from build123d import *

# Parameters (mm, degrees)
BOSS_EXTRUDE1_DEPTH      = 97
BOSS_EXTRUDE1_DEPTH_BACK = 64
SKETCH6_R                = 3
CUT_EXTRUDE1_DEPTH       = 10
SKETCH8_R                = 3
CUT_EXTRUDE3_DEPTH       = 10


with BuildPart() as part:
    # Sketch3 → Boss-Extrude1 (new, two sides: drawn at the far end of the back side and taken through both)
    with BuildSketch(Plane(origin=(-16.16759993, 0, 0), x_dir=(0, 0, -1), z_dir=(1, 0, 0)).offset(-BOSS_EXTRUDE1_DEPTH_BACK)):
        Polygon((746.208968128, 603.456840762), (886.208968128, 603.456840762), (949.708968128, 493.471614481), (923.661741478, 345.75045153), (946.661741478, 345.75045153), (946.661741478, 347.02045153), (925.175268541, 347.02045153), (951.03994149, 493.706300996), (886.94220297, 604.726840762), (745.475733286, 604.726840762), (681.358982713, 493.673371154), (730.060945884, 282.721992649), (731.298395866, 283.007680488), (682.708968128, 493.471614481), align=None)
    extrude(amount=BOSS_EXTRUDE1_DEPTH + BOSS_EXTRUDE1_DEPTH_BACK)

    # Sketch6 → Cut-Extrude1 (cut)
    with BuildSketch(Plane(origin=(0, 347.02045153, 0), x_dir=(1, 0, 0), z_dir=(0, 1, 0))):
        with Locations(Location((-69.5, 935.918505009, 0), (0, 0, 180))):
            Circle(SKETCH6_R)
        with Locations(Location((69.000000001, 935.918505009, 0), (0, 0, 180))):
            Circle(SKETCH6_R)
    extrude(amount=-CUT_EXTRUDE1_DEPTH, mode=Mode.SUBTRACT)

    # Sketch8 → Cut-Extrude3 (cut)
    with BuildSketch(Plane(origin=(0, 174.325401486, -755.08627081), x_dir=(1, 0, 0), z_dir=(0, -0.22495105434386187, 0.9743700647852359))):
        with Locations(Location((69, 160.202749263, 0), (0, 0, 270))):
            Circle(SKETCH8_R)
        with Locations(Location((-69.5, 160.49556469, 0), (0, 0, 270))):
            Circle(SKETCH8_R)
    extrude(amount=-CUT_EXTRUDE3_DEPTH, mode=Mode.SUBTRACT)


solid = part.part
Model file for the job. Use its own axes, mm. A direction names the side the tool comes from. Coordinates: 2 decimals unless noted, no trailing zeros. Loops run counter-clockwise (first coordinate to the right, second up) from the corner with the lowest first, then second, coordinate; pieces in that order, holes last. Notation, with made-up numbers: (62, 41) -> (111, 41) arc R35 cw to (111, 76) -> close; hole circle Ø6 at (78, -17.75). An arc over 180 degrees is marked (long way). Use one line per item in the form item = value. Start each with the question number.
(1) Cut at C-C on x = 22. Give the cut face in (y, z).
(2) Tool access for faces 1 (the flat face through (-1, 603.457, -815)), 2 (the flat face through (-1, 347.02, -936)), 3 (the flat face through (-0.79, 547.69, -714.01)): list every direction of +Z, -Z, +X, -X, +Y, -Y with a clear straight run to the whole face (end or side of a thin tool).
(3) Cut at B-B on y = 400.5. Give the cut face in (x, z), and give its area (3 significant figures).
(4) Cut at A-A on z = -700.5. Give the cut face in (x, y), and give its area (3 significant figures).
(5) Pull direction Z, two halves, no side cores. Call faces 4 (the flat face through (-0.795, 549.977, -713.866)), 5 (the flat face through (-0.795, 549.234, -917.514)), 6 (the flat face through (-1, 345.75, -935)), 7 (the flat face through (-0.795, 386.766, -707.344)): pulls with the +Z half, pulls with the -Z half, needs draft (parallel to the pull), parting line crosses it, or undercut.
(6) Flat gauge pins, fed straight in: pin 1 (8 mm diameter, centred on x = -47, z = -729.5, fed in from +Y); pin 2 (5 mm diameter, centred on x = 69, z = -935.92, fed in from +Y); pin 3 (10 mm diameter, centred on x = -35, z = -770.5, fed in from -Y). Where does each tip first touch, or does it go through?
(7) Cut at D-D on z = -754. Give the cut face in (x, y), and give its area (3 significant figures).
(8) Probe probe 1 along Z at (x, y) = (-69.5, 346.55); probe 2 along Z at (x, y) = (-69, 346); probe 3 along Y at (x, z) = (52.5, -851.5). List the from-to ranges inside material, lowest first. Write a range as from..to.
Values:
q1.outline = (282.72, -730.06) -> (283.01, -731.3) -> (493.47, -682.71) -> (603.46, -746.21) -> (603.46, -886.21) -> (493.47, -949.71) -> (345.75, -923.66) -> (345.75, -946.66) -> (347.02, -946.66) -> (347.02, -925.18) -> (493.71, -951.04) -> (604.73, -886.94) -> (604.73, -745.48) -> (493.67, -681.36) -> close
q2.face_1 = +X, -X, -Y
q2.face_2 = -Z, +X, -X
q2.face_3 = +X, -X
q3.outline = (-80.17, -934.61) -> (80.83, -934.61) -> (80.83, -933.32) -> (-80.17, -933.32) -> close; (-80.17, -704.17) -> (80.83, -704.17) -> (80.83, -702.87) -> (-80.17, -702.87) -> close
q3.area = 417 mm2
q4.outline = (-80.17, 410.76) -> (80.83, 410.76) -> (80.83, 416.41) -> (-80.17, 416.41) -> close; (-80.17, 524.29) -> (80.83, 524.29) -> (80.83, 526.83) -> (-80.17, 526.83) -> close
q4.area = 1,320 mm2
q5.face_4 = pulls with the +Z half
q5.face_5 = undercut
q5.face_6 = needs draft
q5.face_7 = undercut
q6.pin_1 = 583.98
q6.pin_2 = 524.22
q6.pin_3 = 603.46
q7.outline = (-80.17, 603.46) -> (80.83, 603.46) -> (80.83, 604.73) -> (-80.17, 604.73) -> close
q7.area = 204 mm2
q8.probe_1 = -946.66..-938.92, -932.92..-923.8, -716.63..-715.33
q8.probe_2 = -946.66..-938.88, -932.96..-923.71, -716.76..-715.45
q8.probe_3 = 603.46..604.73
